Part model, mm, in its own coordinate system. A direction names the side the tool comes from. Coordinates: 2 decimals unless noted, no trailing zeros. Order: outer loops, then holes, each group sorted by start corner. A loop starts at its lowest first (then second) coordinate and runs counter-clockwise, first axis right, second up.
from build123d import *

# Parameters (mm, degrees)
F1_DEPTH = 165.1
F2_R     = 2.38125
F3_DEPTH = 1.5875
F4_R     = 2.38125
F5_DEPTH = 25.4


with BuildPart() as f1:
    # F0 (on Top) → F1 (new body, symmetric)
    with BuildSketch(Plane.XY):
        Polygon((1.5875, 25.4), (0, 25.4), (0, 0), (25.4, 0), (25.4, 1.5875), (1.5875, 1.5875), align=None)
    extrude(amount=F1_DEPTH, both=True)

    # F2 (on face) → F3 (cut, through all)
    with BuildSketch(Plane(origin=(0, 1.5875, 0), x_dir=(-1, 0, 0), z_dir=(0, 1, 0))):
        with Locations((-12.7, -152.4)):
            Circle(F2_R)
        with Locations((-12.7, 152.4)):
            Circle(F2_R)
        with Locations((-12.7, 76.2)):
            Circle(F2_R)
        with Locations((-12.7, -76.2)):
            Circle(F2_R)
        with Locations((-12.7, 0)):
            Circle(F2_R)
    extrude(amount=-F3_DEPTH, mode=Mode.SUBTRACT)

    # F4 (on face) → F5 (cut)
    with BuildSketch(Plane.YZ.offset(1.5875)):
        with Locations((9.525, -152.4)):
            Circle(F4_R)
        with Locations((9.525, -76.2)):
            Circle(F4_R)
        with Locations((9.525, 0)):
            Circle(F4_R)
        with Locations((9.525, 76.2)):
            Circle(F4_R)
        with Locations((9.525, 152.4)):
            Circle(F4_R)
    extrude(amount=-F5_DEPTH, mode=Mode.SUBTRACT)


solid = f1.part
Q1. Pin check, flat tips, straight feed: pin 1 Ø6 at (x, z) = (12.7, 152.4) entering from +Y; pin 2 Ø8 at (y, z) = (14.5, 32.5) entering from +X. Stop position of each tip, or through.
Results list:
pin 1: stops at y = 1.59
pin 2: stops at x = 1.59
Q2. Which spindle directions (+Z, -Z, +X, -X, +Y, -Y) get a long thin tool onto all of the face, cutting with end or side? Do faces 1 (the face through (1, 7, -165.1)), 2 (the face through (16, 1.588, 2)). Say none if no direction does.
Results list:
face 1: -Z, +X, -X, +Y, -Y
face 2: +Z, -Z, +X, +Y
Q3. Cut at B-B on y = 17.75. Write the cut outline in (x, z), and give its area (3 significant figures).
Results list:
outline: (0, -165.1) - (1.59, -165.1) - (1.59, 165.1) - (0, 165.1) - close
area: 524 mm2
Q4. Wall check: line 1 along Z through (x, y) = (12.7, 0.4); line 2 along Y through (x, z) = (0.7, -152.4); line 3 along X through (y, z) = (18.5, 140). Give the ranges that are in metal, low to high.
Results list:
line 1: z = -165.1 to -154.78, -150.02 to -78.58, -73.82 to -2.38, 2.38 to 73.82, 78.58 to 150.02, 154.78 to 165.1
line 2: y = 0 to 7.14, 11.91 to 25.4
line 3: x = 0 to 1.59
Q5. Cut at A-A on z = -120. Write the cut outline in (x, y), and give its area (3 significant figures).
Results list:
outline: (0, 0) - (25.4, 0) - (25.4, 1.59) - (1.59, 1.59) - (1.59, 25.4) - (0, 25.4) - close
area: 78.1 mm2
